Autodesk Inventor part; units mm, degrees
ref_plane "XZ Plane" through (0, 0, 0) normal (0, 1, 0) x (-1, 0, 0)
sketch "Szkic1" plane through (0, 0, 0) normal (0, 1, 0) x (-1, 0, 0)
  circle A0 centre (0, 0) radius 1.75
  dimension "d0" = 3.5
extrude "Wyciągnięcie proste1" add sketch "Szkic1" along normal blind 7
sketch "Szkic2" plane through (0, 7, 0) normal (0, 1, 0) x (1, 0, 0)
  circle A0 centre (0, 0) radius 3
  dimension "d3" = 6
extrude "Wyciągnięcie proste2" add sketch "Szkic2" along normal blind 50
sketch "Szkic3" plane through (0, 57, 0) normal (0, 1, 0) x (1, 0, 0)
  circle A0 centre (0, 0) radius 1.75
  circle A1 centre (0, 0) radius 1.75
  dimension "d6" = 3.5
extrude "Wyciągnięcie proste3" add sketch "Szkic3" along normal blind 7
properties part number "rod"
Verification items for the finished model (mm, model axes). A direction names the side the tool comes from. Round coordinates to 2 decimals unless told otherwise and drop trailing zeros. Order: outer loops, then holes, each group sorted by start corner. A loop starts at its lowest first (then second) coordinate and runs counter-clockwise, first axis right, second up.
1. Section check A-A on x = 0. Record the cut outline in (y, z), then the cut area to 3 significant figures.
Final values:
outline: (0, -1.75) - (7, -1.75) - (7, -3) - (57, -3) - (57, -1.75) - (64, -1.75) - (64, 1.75) - (57, 1.75) - (57, 3) - (7, 3) - (7, 1.75) - (0, 1.75) - close
area: 349 mm2
2. Thickness scan on L1, parallel to Y at x = -0.25, z = 2.45; L2, parallel to Z at x = 0.25, y = 46.5; L3, parallel to X at y = 23, z = -1.6. Record the ranges inside material, lowest first.
Final values:
L1: y = 7 to 57
L2: z = -2.99 to 2.99
L3: x = -2.54 to 2.54
3. Section check C-C on y = 17.5. Record the cut outline in (x, z), then the cut area to 3 significant figures.
Final values:
outline: circle Ø6 at (0, 0)
area: 28.3 mm2
4. Access from +Z, -Z, +X, -X, +Y, -Y to the whole of each face (thin tool, end or side, straight path). Record for faces 1 (the cylindrical face through (-3, 32, 0)), 2 (the cylindrical face through (1.617, 60.451, -0.67)), 3 (the cylindrical face through (-1.617, 3.451, 0.67)).
Final values:
face 1: +Y, -Y
face 2: +Y
face 3: -Y
5. Section check B-B on z = 0. Record the cut outline in (x, y).
Final values:
outline: (-3, 7) - (-1.75, 7) - (-1.75, 0) - (1.75, 0) - (1.75, 7) - (3, 7) - (3, 57) - (1.75, 57) - (1.75, 64) - (-1.75, 64) - (-1.75, 57) - (-3, 57) - close
